Could you check a few things on this model? Use its own coordinates, in mm. Round coordinates to 2 decimals unless told otherwise and drop trailing zeros. Loops run counter-clockwise (first coordinate to the right, second up) from the corner with the lowest first, then second, coordinate; pieces in that order, holes last. Notation, with made-up numbers: M -28.5,-10.75 L -8.5,-10.75 A13 cw -8.5,-2.75 Z; hole C 54,32.25 d2. An arc over 180 degrees is marked long. Answer in a Markdown table with one row per item.
```python
from build123d import *

# Parameters (mm, degrees)
BOSS_EXTRUDE1_DEPTH = 3.175
FILLET1_R           = 12.7


with BuildPart() as part:
    # Sketch1 → Boss-Extrude1 (new body)
    with BuildSketch(Plane(origin=(0, 407.886507076, 975.028347662), x_dir=(1, 0, 0), z_dir=(0, 0.38592481598359657, 0.922530236040005))):
        Polygon((144.331189968, 73.343707369), (-144.331189968, 72.063414553), (-110.678400742, -322.378637797), (110.678400742, -319.252822954), align=None)
    extrude(amount=-BOSS_EXTRUDE1_DEPTH)

    # Fillet1
    fillet1_edges = [part.edges().sort_by_distance(p)[0] for p in [
        (110.678400742, 112.753469314, 1096.771417863),
        (-110.678400742, 109.86981061, 1097.977747381),
        (-144.331189968, 473.754530268, 945.752770911),
        (144.331189968, 474.935639101, 945.258674142),
    ]]
    fillet(fillet1_edges, radius=FILLET1_R)


solid = part.part
```
1) I want a section at B-B, the plane z = 979. Please give me the cut outline in (x, y), plus the area to 3 significant figures.
Computed:
| item | result |
|---|---|
| outline | M -137.3,398.39 L -136.66,390.17 L 136.51,390.17 L 137.16,398.39 Z |
| area | 2,250 mm² |
2) I want a section at A-A, the plane x = 81.5. Please give me the cut outline in (y, z), plus the area to 3 significant figures.
Computed:
| item | result |
|---|---|
| outline | M 111.76,1095.47 L 474.07,943.9 L 475.29,946.83 L 112.99,1098.39 Z |
| area | 1,250 mm² |
3) I need wall thicknesses on line 1 (Z direction, x = 5, y = 370); line 2 (Z direction, x = -96.5, y = 409.5); line 3 (Y direction, x = 57.5, z = 1024). Which ranges of each line are inside material? Lowest first, please.
Computed:
| item | result |
|---|---|
| line 1 | z = 987.44 to 990.88 |
| line 2 | z = 970.91 to 974.35 |
| line 3 | y = 282.6 to 290.82 |
4) Will these pins go through, and if not, where does the flat tip stop? P1, Ø3, axis at x = -4, z = 1079.5, coming from the +Y side; P2, Ø1.5, axis at x = 73, z = 988, coming from the -Y side; P3, Ø6, axis at x = -16, z = 1064, coming from the +Y side.
Computed:
| item | result |
|---|---|
| P1 | stops at y = 161.74 |
| P2 | stops at y = 366.86 |
| P3 | stops at y = 202.38 |
